The listing builds one solid part. Answer for the finished solid, in the listing's coordinates (mm). Face numbers are marked on the shaded views. Coordinates: 2 decimals unless noted, no trailing zeros. Order: outer loops, then holes, each group sorted by start corner. A loop starts at its lowest first (then second) coordinate and runs counter-clockwise, first axis right, second up. Notation, with made-up numbers: (-21.75, 41) - (-6.75, 41) arc R21 ccw to (-6.75, 69) - close; hole circle Ø7 at (-31, 49). An arc over 180 degrees is marked (long way). Use a Markdown table: item, result. Add a question column.
Item 1: Flat-ended cylindrical pins translate along their axes: P1, Ø1.5, axis at x = -29.5, y = 18.5, coming from the -Z side; P2, Ø5, axis at x = 0, z = 33.34, coming from the +Y side; P3, Ø4, axis at x = -4, y = 26.5, coming from the +Z side; P4, Ø3, axis at x = 35, z = -2.5, coming from the -Y side. Find the tip coordinate at first contact, or state that the pin passes through.
Item 2: The part is cut by section D-D, the plane z = 0. Give the vertices of the cut face in (x, y), then the cut area to 3 significant figures.
Item 3: The part is cut by section B-B, the plane z = 31.5. Give the vertices of the cut face in (x, y).
Item 4: The mould has two halves that part along Z. Classify the marked faces 1, 2 and 3: released by +Z, released by -Z, zero draft, split by the parting line, or undercut.
Item 5: Find the intervals of material crossed by line 1 along X through (y, z) = (33, 0); line 2 along Z through (x, y) = (1, 15.5); line 3 along Y through (x, z) = (-27, 12), in increasing order.
Item 6: The part is cut by section A-A, the plane x = 0. Give the vertices of the cut face in (y, z), then the cut area to 3 significant figures.
Item 7: The part is cut by section C-C, the plane x = 20. Give the vertices of the cut face in (y, z), then the cut area to 3 significant figures.
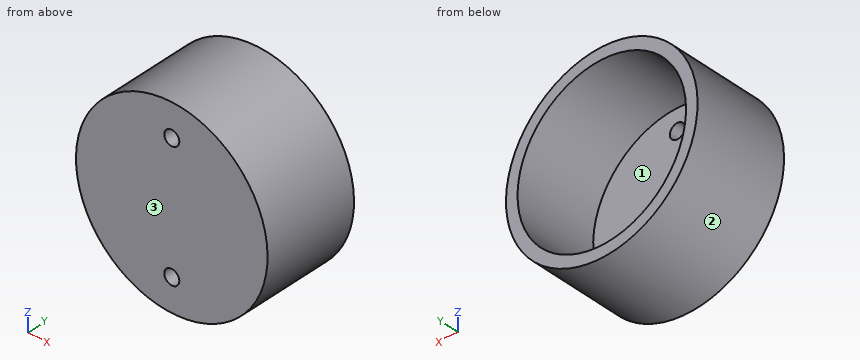
from build123d import *

# Parameters (mm, degrees)
SKETCH1_R           = 50.546
BOSS_EXTRUDE1_DEPTH = 50.8
SKETCH2_R           = 44.45
CUT_EXTRUDE1_DEPTH  = 44.45
SKETCH3_R           = 3.96875
CUT_EXTRUDE2_DEPTH  = 44.45


with BuildPart() as part:
    # Sketch1 → Boss-Extrude1 (new body)
    with BuildSketch(Plane(origin=(0, 0, 0), x_dir=(1, 0, 0), z_dir=(0, 1, 0))):
        with Locations(Location((0, 0, 0), (0, 0, 270))):
            Circle(SKETCH1_R)
    extrude(amount=BOSS_EXTRUDE1_DEPTH)

    # Sketch2 → Cut-Extrude1 (cut)
    with BuildSketch(Plane(origin=(0, 50.8, 0), x_dir=(1, 0, 0), z_dir=(0, 1, 0))):
        with Locations(Location((0, 0, 0), (0, 0, 270))):
            Circle(SKETCH2_R)
    extrude(amount=-CUT_EXTRUDE1_DEPTH, mode=Mode.SUBTRACT)

    # Sketch3 → Cut-Extrude2 (cut)
    with BuildSketch(Plane.XZ):
        with Locations(Location((0, 33.3375, 0), (0, 0, 270))):
            Circle(SKETCH3_R)
        with Locations(Location((0, -33.3375, 0), (0, 0, 270))):
            Circle(SKETCH3_R)
    extrude(amount=-CUT_EXTRUDE2_DEPTH, mode=Mode.SUBTRACT)


solid = part.part
Solution:
| question | item | result |
|---|---|---|
| 1 | P1 | stops at z = -41.57 |
| 1 | P2 | passes through |
| 1 | P3 | stops at z = 50.51 |
| 1 | P4 | stops at y = 0 |
| 2 | outline | (-50.55, 0) - (50.55, 0) - (50.55, 50.8) - (44.45, 50.8) - (44.45, 6.35) - (-44.45, 6.35) - (-44.45, 50.8) - (-50.55, 50.8) - close |
| 2 | area | 1,180 mm2 |
| 3 | outline | (-39.53, 0) - (-3.52, 0) - (-3.52, 6.35) - (-31.36, 6.35) - (-31.36, 50.8) - (-39.53, 50.8) - close; (3.52, 0) - (39.53, 0) - (39.53, 50.8) - (31.36, 50.8) - (31.36, 6.35) - (3.52, 6.35) - close |
| 4 | face 1 | undercut |
| 4 | face 2 | split by the parting line |
| 4 | face 3 | zero draft |
| 5 | line 1 | x = -50.55 to -44.45, 44.45 to 50.55 |
| 5 | line 2 | z = -50.54 to -44.44, 44.44 to 50.54 |
| 5 | line 3 | y = 0 to 6.35 |
| 6 | outline | (0, -50.55) - (50.8, -50.55) - (50.8, -44.45) - (6.35, -44.45) - (6.35, -37.31) - (0, -37.31) - close; (0, -29.37) - (6.35, -29.37) - (6.35, 29.37) - (0, 29.37) - close; (0, 37.31) - (6.35, 37.31) - (6.35, 44.45) - (50.8, 44.45) - (50.8, 50.55) - (0, 50.55) - close |
| 6 | area | 1,080 mm2 |
| 7 | outline | (0, -46.42) - (50.8, -46.42) - (50.8, -39.7) - (6.35, -39.7) - (6.35, 39.7) - (50.8, 39.7) - (50.8, 46.42) - (0, 46.42) - close |
| 7 | area | 1,190 mm2 |
